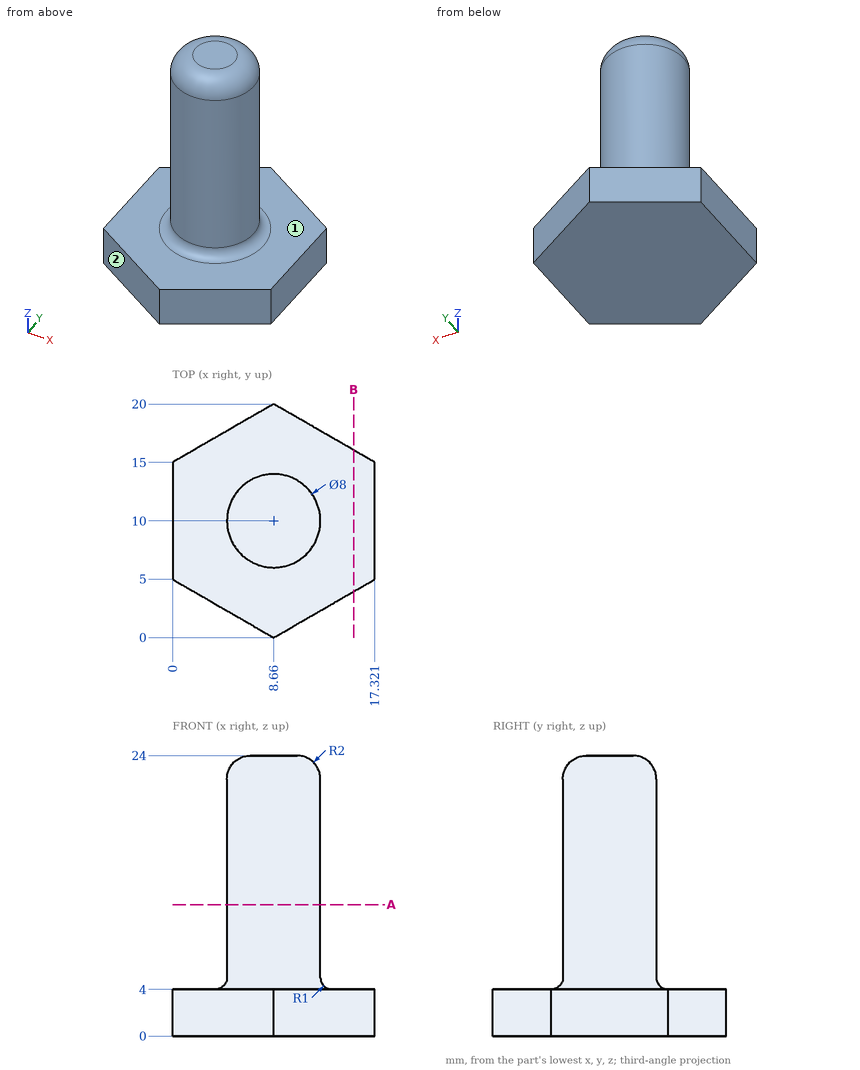
Source: three-view drawing plus pictorial views. Frame: mm from the lowest corner of the part. A direction names the side the tool comes from. Round coordinates to 2 decimals unless told otherwise and drop trailing zeros. Order: outer loops, then holes, each group sorted by start corner. A loop starts at its lowest first (then second) coordinate and runs counter-clockwise, first axis right, second up. Notation, with made-up numbers: (37, 13.25) -> (59, 13.25) arc R18 cw to (59, 20.25) -> close; hole circle Ø11 at (-10.75, -21.5). An arc over 180 degrees is marked (long way). Use one line per item in the form item = value.
(1) Section A-A on z = 11.25. Return loops of the section in (x, y).
Results list:
outline = circle Ø8 at (8.66, 10)
(2) Access query for the marked faces 1 and 2. Directions: +Z, -Z, +X, -X, +Y, -Y. A direction counts if a zero-diameter tool reaches every point of the face in a straight line with its end or side. Return the directions, or none.
Results list:
face_1 = +Z
face_2 = +Z, -Z, -X, -Y
(3) Ray query, probe 1 along Z at (x, y) = (3, 4); probe 2 along Y at (x, z) = (8.5, 11.25); probe 3 along Y at (x, z) = (5, 4.5) (1 decimal). Return the intervals inside material, ascending. Write a range as [from, to].
Results list:
probe_1 = [0, 4]
probe_2 = [6, 14]
probe_3 = [8.1, 11.9]
(4) First-contact query: pin 1 Ø6 at (x, z) = (11, 16.5) entering from -Y; pin 2 Ø2 at (x, y) = (5, 6) entering from +Z (1 decimal); pin 3 Ø2 at (x, y) = (7.5, 15.5) entering from +Z (1 decimal). Flat tips, straight axial feed; report the tip coordinate or a pass-through.
Results list:
pin_1 = 6
pin_2 = 4.2
pin_3 = 4.1
(5) Section B-B on x = 15.5. Return loops of the section in (y, z).
Results list:
outline = (3.95, 0) -> (16.05, 0) -> (16.05, 4) -> (3.95, 4) -> close
